from build123d import *

# Parameters (mm, degrees)
BOSS_EXTRUDE1_DEPTH = 1.4986
MIRROR1_START       = -139.7
MIRROR1_OUTLINE_W   = 101.6
MIRROR1_OUTLINE_H   = 2.9972
MIRROR1_DEPTH       = 279.4
MIRROR1_START_2     = -145.288
MIRROR1_2_OUTLINE_W = 40.770628572
MIRROR1_2_OUTLINE_H = 2.9972
MIRROR1_2_DEPTH     = 5.588
MIRROR1_START_3     = -97.79
MIRROR1_3_OUTLINE_W = 2.9972
MIRROR1_3_OUTLINE_H = 2.9972
MIRROR1_3_DEPTH     = 47.498
MIRROR1_START_4     = -2.794
MIRROR1_4_OUTLINE_W = 2.9972
MIRROR1_4_OUTLINE_H = 2.9972
MIRROR1_4_DEPTH     = 47.498
MIRROR1_START_5     = 92.202
MIRROR1_5_OUTLINE_W = 2.9972
MIRROR1_5_OUTLINE_H = 2.9972
MIRROR1_5_DEPTH     = 47.498
CUT_EXTRUDE2_DEPTH  = 204.666583022


# Read off the part's stored shape, not the designer's step: Mirror1
with BuildPart() as part:
    # Sketch1 → Boss-Extrude1 (new, symmetric)
    with BuildSketch(Plane.XY):
        Polygon((-38.1, 139.7), (-142.6972, 139.7), (-142.6972, 92.202), (-139.7, 92.202), (-139.7, 44.704), (-142.6972, 44.704), (-142.6972, -2.794), (-139.7, -2.794), (-139.7, -50.292), (-142.6972, -50.292), (-142.6972, -97.79), (-139.7, -97.79), (-139.7, -139.7), (-101.926571429, -139.7), (-101.926571429, -145.288), (-61.155942857, -145.288), (-61.155942857, -139.7), (-38.1, -139.7), align=None)
    extrude(amount=BOSS_EXTRUDE1_DEPTH, both=True)

    # Mirror1 outline → Mirror1 (add)
    with BuildSketch(Plane(origin=(0, 0, 0), x_dir=(1, 0, 0), z_dir=(0, 1, 0)).offset(MIRROR1_START)):
        with Locations((12.7, 0)):
            Rectangle(MIRROR1_OUTLINE_W, MIRROR1_OUTLINE_H)
    extrude(amount=MIRROR1_DEPTH)

    # Mirror1 2 outline → Mirror1 2 (add)
    with BuildSketch(Plane(origin=(0, 0, 0), x_dir=(1, 0, 0), z_dir=(0, 1, 0)).offset(MIRROR1_START_2)):
        with Locations((5.341257143, 0)):
            Rectangle(MIRROR1_2_OUTLINE_W, MIRROR1_2_OUTLINE_H)
    extrude(amount=MIRROR1_2_DEPTH)

    # Mirror1 3 outline → Mirror1 3 (add)
    with BuildSketch(Plane(origin=(0, 0, 0), x_dir=(1, 0, 0), z_dir=(0, 1, 0)).offset(MIRROR1_START_3)):
        with Locations((64.9986, 0)):
            Rectangle(MIRROR1_3_OUTLINE_W, MIRROR1_3_OUTLINE_H)
    extrude(amount=MIRROR1_3_DEPTH)

    # Mirror1 4 outline → Mirror1 4 (add)
    with BuildSketch(Plane(origin=(0, 0, 0), x_dir=(1, 0, 0), z_dir=(0, 1, 0)).offset(MIRROR1_START_4)):
        with Locations((64.9986, 0)):
            Rectangle(MIRROR1_4_OUTLINE_W, MIRROR1_4_OUTLINE_H)
    extrude(amount=MIRROR1_4_DEPTH)

    # Mirror1 5 outline → Mirror1 5 (add)
    with BuildSketch(Plane(origin=(0, 0, 0), x_dir=(1, 0, 0), z_dir=(0, 1, 0)).offset(MIRROR1_START_5)):
        with Locations((64.9986, 0)):
            Rectangle(MIRROR1_5_OUTLINE_W, MIRROR1_5_OUTLINE_H)
    extrude(amount=MIRROR1_5_DEPTH)

    # Sketch2<3> → Cut-Extrude2 (cut, through all)
    with BuildSketch(Plane.XY.offset(1.4986)):
        Polygon((66.4972, 139.7), (-38.1, 139.7), (-38.1, -139.7), (-15.044057143, -139.7), (-15.044057143, -145.288), (25.726571429, -145.288), (25.726571429, -139.7), (63.5, -139.7), (63.5, -97.79), (66.4972, -97.79), (66.4972, -50.292), (63.5, -50.292), (63.5, -2.794), (66.4972, -2.794), (66.4972, 44.704), (63.5, 44.704), (63.5, 92.202), (66.4972, 92.202), align=None)
    extrude(amount=-CUT_EXTRUDE2_DEPTH, mode=Mode.SUBTRACT)


solid = part.part
Source: CAD feature listing. Evaluate the final solid. Frame: model axes, mm. Round coordinates to 2 decimals unless told otherwise and drop trailing zeros. Write each loop counter-clockwise with the first axis right and the second up, starting at its lowest first coordinate (ties: lowest second). Pieces come first, ordered by that corner, then holes. Notation, with made-up numbers: (-14.5, 44.25) - (0.5, 44.25) arc R32 cw to (0.5, 72.25) - close; hole circle Ø1 at (-36, 30.5). An arc over 180 degrees is marked (long way). Use CSV: the item, a comma, the result in double quotes. Start each with the question number.
(1) Cut plane C-C, the plane x = -120.5. Return loops of the section in (y, z), and give its area (3 significant figures).
(2) Cut plane B-B, the plane y = -16. Return loops of the section in (x, z).
(3) Cut plane A-A, the plane z = 0.1. Return loops of the section in (x, y), and give its area (3 significant figures).
(4) Material intervals for probe 1 along Y at (x, z) = (-103.5, 0.55); probe 2 along X at (y, z) = (-34.5, -1), sorted ascending. Write a range as [from, to].
(5) First-contact query: pin 1 Ø1.5 at (y, z) = (-141.5, 0.5) entering from +X; pin 2 Ø1.5 at (x, z) = (-142, -0.5) entering from -Y; pin 3 Ø0.9 at (y, z) = (-141.5, -0.5) entering from -X. Flat tips, straight axial feed; report the tip coordinate or a pass-through.
Geometry says:
1,outline,"(-139.7, -1.5) - (139.7, -1.5) - (139.7, 1.5) - (-139.7, 1.5) - close"
1,area,"837 mm²"
2,outline,"(-139.7, -1.5) - (-38.1, -1.5) - (-38.1, 1.5) - (-139.7, 1.5) - close"
3,outline,"(-142.7, -97.79) - (-139.7, -97.79) - (-139.7, -139.7) - (-101.93, -139.7) - (-101.93, -145.29) - (-61.16, -145.29) - (-61.16, -139.7) - (-38.1, -139.7) - (-38.1, 139.7) - (-142.7, 139.7) - (-142.7, 92.2) - (-139.7, 92.2) - (-139.7, 44.7) - (-142.7, 44.7) - (-142.7, -2.79) - (-139.7, -2.79) - (-139.7, -50.29) - (-142.7, -50.29) - close"
3,area,"29,000 mm²"
4,probe 1,"[-139.7, 139.7]"
4,probe 2,"[-139.7, -38.1]"
5,pin 1,"x = -61.16"
5,pin 2,"y = -97.79"
5,pin 3,"x = -101.93"
